Autodesk Inventor part; units mm, degrees
ref_plane "YZ Plane" through (0, 0, 0) normal (1, 0, 0) x (0, 1, 0)
ref_plane "XZ Plane" through (0, 0, 0) normal (0, 1, 0) x (-1, 0, 0)
ref_plane "XY Plane" through (0, 0, 0) normal (0, 0, 1) x (1, 0, 0)
sketch "Sketch1" plane through (0, 0, 0) normal (0, 0, 1) x (1, 0, 0)
  line L0 (-40, 0) -> (-40, 14.0559)
  line L1 (-42, 14.0559) -> (-42, -2)
  line L2 (-40, 0) -> (0, 0)
  line L3 (0, 0) -> (0, -2)
  line L4 (0, -2) -> (-42, -2)
  line L5 (0, -5.2112) -> (0, 17.2671)
  line L6 (-42, 14.0559) -> (-40, 14.0559)
  dimension "d5" = 2
  dimension "radius" = 40
  dimension "d7" = 2
revolve "Revolution1" add sketch "Sketch1" angle 360 about axis through (0, -10, 0) along (0, 1, 0)
sketch "Sketch4" plane through (0, 0, 0) normal (0, 0, 1) x (1, 0, 0)
  line L0 (40.24, 12) -> (-40.24, 12)
  line L1 (0, 0) -> (0, 6)
  line L2 (0, 6) -> (0, 12)
hole "Hole3" at (0, 6, 0) direction (0, 0, -1) diameter 7 end through all both
equation "\"d30\" = PenetrationUpstreamInnerDiameter + 2 * PenetrationUpstreamThickness"
equation "\"d5\" = thickness"
equation "\"radius\" = 0.5 * SaltDiameter"
equation "\"d7\" = thickness"
equation "\"thickness\" = crucible_thickness"
equation "\"CrucibleHeightBelowMembrane\" = 14"
properties part number "UpstreamVolume"
Can you work these out from the model? Positions are in its coordinate system, mm. A direction names the side the tool comes from. Give positions to 0.01 mm unless a question says otherwise; leave off trailing zeros. Loops run counter-clockwise (first coordinate to the right, second up) from the corner with the lowest first, then second, coordinate; pieces in that order, holes last. Notation, with made-up numbers: M 17.25,84 L 42.25,84 A34 cw 42.25,118 Z; hole C 31,-32 d8. An arc over 180 degrees is marked long. One line per item, written item: value.
(1) We'd pull the mould along X, two halves only. Please class faces 3 (the face through (-40.06, 5.92, -12.62)), 4 (the face through (-37.1, 14.056, -15.4)), 5 (the face through (-3.47, 6.46, -40.94)): released by +X, released by -X, zero draft, split by the parting line, or undercut.
Returned:
face 3: split by the parting line
face 4: zero draft
face 5: undercut
(2) I need wall thicknesses on line 1 (Y direction, x = 0, z = 41); line 2 (Y direction, x = -8, z = -20); line 3 (Z direction, x = -11.5, y = 5.25). Which ranges of each line are inside material? Lowest first, please.
Returned:
line 1: -2 to 2.5, 9.5 to 14.06
line 2: -2 to 0
line 3: -40.39 to -38.31, 38.31 to 40.39
(3) Suppose I cut it at A-A on x = 0. List the corners of the cut face in (y, z) for me.
Returned:
outline: M -2,-42 L 2.5,-42 L 2.5,-40 L 0,-40 L 0,40 L 2.5,40 L 2.5,42 L -2,42 Z; M 9.5,-42 L 14.06,-42 L 14.06,-40 L 9.5,-40 Z; M 9.5,40 L 14.06,40 L 14.06,42 L 9.5,42 Z
(4) Will these pins go through, and if not, where does the flat tip stop? pin 1 (2 mm diameter, centred on x = -7.5, z = 28, fed in from +Y); pin 2 (5 mm diameter, centred on x = -32, y = 8.5, fed in from -Z); pin 3 (5 mm diameter, centred on y = 3, z = 28.5, fed in from +X).
Returned:
pin 1: y = 0
pin 2: z = -29.9
pin 3: x = 32.98
(5) Which directions (+Z, -Z, +X, -X, +Y, -Y) give clear straight access to the entire face, cutting with the end or side of a thin tool? Please do faces 1 (the face through (1, 0, 1)), 2 (the face through (1, -2, 1)).
Returned:
face 1: +Y
face 2: +Z, -Z, +X, -X, -Y
(6) Suppose I cut it at D-D on x = 35. List the corners of the cut face in (y, z) for me, plus the area to 3 significant figures.
Returned:
outline: M -2,-23.22 L 14.06,-23.22 L 14.06,-19.36 L 0,-19.36 L 0,19.36 L 14.06,19.36 L 14.06,23.22 L -2,23.22 Z
area: 201 mm^2
(7) Suppose I cut it at C-C on z = 0. List the corners of the cut face in (x, y) for me.
Returned:
outline: M -42,-2 L 42,-2 L 42,14.06 L 40,14.06 L 40,0 L -40,0 L -40,14.06 L -42,14.06 Z
